Verification items for the finished model (mm, model axes). A direction names the side the tool comes from. Coordinates: 2 decimals unless noted, no trailing zeros. Write each loop counter-clockwise with the first axis right and the second up, starting at its lowest first coordinate (ties: lowest second). Pieces come first, ordered by that corner, then holes. Notation, with made-up numbers: (-9, -38) -> (12, -38) arc R14 cw to (12, -19) -> close; hole circle Ø7 at (77.25, -8.75). An arc over 180 degrees is marked (long way). Use a Markdown table: item, result. Add a question column.
from build123d import *

# Parameters (mm, degrees)
BOSS_EXTRUDE1_DEPTH = 30


with BuildPart() as part:
    # Sketch2 → Boss-Extrude1 (new body)
    with BuildSketch(Plane(origin=(0, 0, 0), x_dir=(1, 0, 0), z_dir=(0, 1, 0))):
        with BuildLine():
            Line((0, 0), (0, 15))
            Line((0, 15), (9.999999101, 15))
            ThreePointArc((9.999999101, 15), (17.5, 22.5), (9.999999101, 30))
            Line((9.999999101, 30), (0, 30))
            Line((0, 30), (0, 55))
            Line((0, 55), (9.999999101, 55))
            ThreePointArc((9.999999101, 55), (17.5, 62.5), (9.999999101, 70))
            Line((9.999999101, 70), (0, 70))
            Line((0, 70), (0, 85))
            Line((0, 85), (10, 85))
            Line((10, 85), (10, 75))
            ThreePointArc((10, 75), (22.5, 62.5), (10, 50))
            Line((10, 50), (10, 35))
            ThreePointArc((10, 35), (22.5, 22.5), (10, 10))
            Line((10, 10), (10, 0))
            Line((10, 0), (0, 0))
        make_face()
    extrude(amount=BOSS_EXTRUDE1_DEPTH)


solid = part.part
1) Cross-section at A-A on x = 5.5. Record the boundary of the cut face in (y, z).
2) Thickness scan on L1, parallel to Z at x = 2, y = 11.25; L2, parallel to Z at x = 16, y = 13.25; L3, parallel to X at y = 5.5, z = -42. Record the ranges inside material, lowest first.
3) Set-up check for faces 1 (the face through (10, 15, -80)), 2 (the face through (10, 15, -43)), 3 (the face through (5, 15, -30)), 4 (the face through (10, 15, -5)), 5 (the face through (5, 15, -85)): record each of +Z, -Z, +X, -X, +Y, -Y from which the full face is reachable in a straight line by a thin tool's end or side.
4) Cross-section at C-C on y = 20.25. Record the boundary of the cut face in (x, z).
5) Cross-section at D-D on z = -22.5. Record the boundary of the cut face in (x, y), then the cut area to 3 significant figures.
6) Cross-section at B-B on x = 12. Record the boundary of the cut face in (y, z), then the cut area to 3 significant figures.
7) Release check for a two-part mould opening along Z. For faces 6 (the face through (0, 15, -7)), 7 (the face through (22.497, 14.79, -62.775)), 8 (the face through (5, 15, 0)) record: released by +Z, released by -Z, zero draft, split by the parting line, or undercut.
8) Gauge pin test, flat ends, axial feed: pin 1 (1 mm diameter, centred on x = 17, y = 10.5, fed in from -Z); pin 2 (5 mm diameter, centred on y = 17, z = -5.5, fed in from +X); pin 3 (10 mm diameter, centred on x = 17.5, y = 20.5, fed in from -Z). Record the tip position at first contact, or that the pin passes through.
Returned:
| question | item | result |
|---|---|---|
| 1 | outline | (0, -85) -> (30, -85) -> (30, -70) -> (0, -70) -> close; (0, -55) -> (30, -55) -> (30, -30) -> (0, -30) -> close; (0, -15) -> (30, -15) -> (30, 0) -> (0, 0) -> close |
| 2 | L1 | z = -85 to -70, -55 to -30, -15 to 0 |
| 2 | L2 | z = -73.47 to -67, -58 to -51.53, -33.47 to -27, -18 to -11.53 |
| 2 | L3 | x = 0 to 10 |
| 3 | face 1 | -Z, +X, +Y, -Y |
| 3 | face 2 | +X, +Y, -Y |
| 3 | face 3 | -X, +Y, -Y |
| 3 | face 4 | +Z, +X, +Y, -Y |
| 3 | face 5 | -Z, +X, -X, +Y, -Y |
| 4 | outline | (0, -85) -> (10, -85) -> (10, -75) arc R12.5 ccw to (10, -50) -> (10, -35) arc R12.5 ccw to (10, -10) -> (10, 0) -> (0, 0) -> (0, -15) -> (10, -15) arc R7.5 cw to (10, -30) -> (0, -30) -> (0, -55) -> (10, -55) arc R7.5 cw to (10, -70) -> (0, -70) -> close |
| 5 | outline | (17.5, 0) -> (22.5, 0) -> (22.5, 30) -> (17.5, 30) -> close |
| 5 | area | 150 mm² |
| 6 | outline | (0, -74.84) -> (30, -74.84) -> (30, -69.73) -> (0, -69.73) -> close; (0, -55.27) -> (30, -55.27) -> (30, -50.16) -> (0, -50.16) -> close; (0, -34.84) -> (30, -34.84) -> (30, -29.73) -> (0, -29.73) -> close; (0, -15.27) -> (30, -15.27) -> (30, -10.16) -> (0, -10.16) -> close |
| 6 | area | 613 mm² |
| 7 | face 6 | zero draft |
| 7 | face 7 | undercut |
| 7 | face 8 | released by +Z |
| 8 | pin 1 | stops at z = -73.18 |
| 8 | pin 2 | stops at x = 10 |
| 8 | pin 3 | stops at z = -74.75 |
